Input: part model. Units: mm. Frame: model coordinates. Give positions to 0.01 mm unless a question says otherwise; leave off trailing zeros. Use a Markdown table: item, result. Add a question column.
from build123d import *

# Parameters (mm, degrees)
SKETCH_1_W      = 10
SKETCH_1_H      = 10
EXTRUDE_1_DEPTH = 10


with BuildPart() as part:
    # Эскиз1 → Бобышка-Вытянуть1 (new body)
    with BuildSketch(Plane(origin=(0, 0, 0), x_dir=(1, 0, 0), z_dir=(0, 1, 0))):
        Polygon((-450, 5), (-450, 15), (-460, 15), (-460, 25), (-450, 25), (450, 25), (460, 25), (460, 15), (450, 15), (450, 5), (460, 5), (460, -5), (450, -5), (450, -15), (460, -15), (460, -25), (450, -25), (-450, -25), (-460, -25), (-460, -15), (-450, -15), (-450, -5), (-460, -5), (-460, 5), align=None)
        with Locations((-415, -10)):
            Rectangle(SKETCH_1_W, SKETCH_1_H, mode=Mode.SUBTRACT)
        with Locations((-415, 10)):
            Rectangle(SKETCH_1_W, SKETCH_1_H, mode=Mode.SUBTRACT)
        with Locations((415, 10)):
            Rectangle(SKETCH_1_W, SKETCH_1_H, mode=Mode.SUBTRACT)
        with Locations((415, -10)):
            Rectangle(SKETCH_1_W, SKETCH_1_H, mode=Mode.SUBTRACT)
    extrude(amount=EXTRUDE_1_DEPTH)


solid = part.part
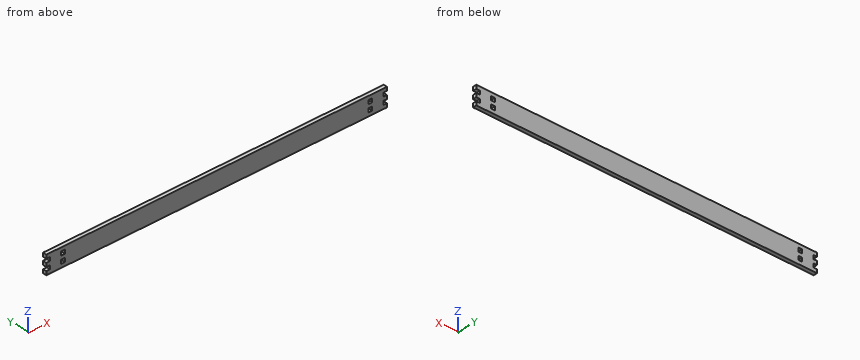
1) Contact query for flat-ended pins moving along their axis: P1, Ø3, axis at y = 5.5, z = -8, coming from the +X side; P2, Ø4, axis at y = 1, z = -5.5, coming from the -X side; P3, Ø5, axis at y = 2.5, z = 9.5, coming from the -X side. Output: stop coordinate, or through.
2) Section query A-A, the plane y = 7.5. State how many separate pieces and enclosed holes the cut face has, and give its area (3 significant figures).
3) Ray query, line 1 (X direction, y = 5.75, z = 13). Return the intervals inside material, ascending. Write a range as [from, to].
Entries:
| question | item | result |
|---|---|---|
| 1 | P1 | stops at x = 450 |
| 1 | P2 | stops at x = -460 |
| 1 | P3 | stops at x = -450 |
| 2 | separate pieces | 1 |
| 2 | enclosed holes | 4 |
| 2 | area | 45,200 mm² |
| 3 | line 1 | x = [-450, -420], [-410, 410], [420, 450] |
